```python
from build123d import *

# Parameters (mm, degrees)
SKETCH_R          = 1.6
PAD_DEPTH         = 6
SKETCH001_R       = 3
POCKET_DEPTH      = 40.001
POCKET_DEPTH_BACK = 40.001


with BuildPart() as toolbody:
    # Sketch → Pad (new body)
    with BuildSketch(Plane.XY):
        Polygon((46, -40), (0, -40), (0, -25), (17.5, -25), (0, -7.5), (0, 7.5), (0, 20), (10, 20), (10, 40), (46, 40), (56, 40), (56, -40), align=None)
        with Locations((53, 0)):
            Circle(SKETCH_R, mode=Mode.SUBTRACT)
        with Locations((53, 35)):
            Circle(SKETCH_R, mode=Mode.SUBTRACT)
        with Locations((53, -35)):
            Circle(SKETCH_R, mode=Mode.SUBTRACT)
        with Locations((39, 35)):
            Circle(SKETCH_R, mode=Mode.SUBTRACT)
        with Locations((39, 0)):
            Circle(SKETCH_R, mode=Mode.SUBTRACT)
        with Locations((39, -35)):
            Circle(SKETCH_R, mode=Mode.SUBTRACT)
        with Locations((15, 35)):
            Circle(SKETCH_R, mode=Mode.SUBTRACT)
        with Locations((15, -35)):
            Circle(SKETCH_R, mode=Mode.SUBTRACT)
        Polygon((15, 0), (28.75, 13.75), (28.75, -13.75), align=None, mode=Mode.SUBTRACT)
    extrude(amount=-PAD_DEPTH)

    # Sketch001 → Pocket (cut, two sides)
    with BuildSketch(Plane.XZ) as pocket_sk:
        with Locations((46, 0)):
            Circle(SKETCH001_R)
    extrude(amount=-POCKET_DEPTH, mode=Mode.SUBTRACT)
    extrude(pocket_sk.sketch, amount=POCKET_DEPTH_BACK, mode=Mode.SUBTRACT)


with BuildPart() as toolfusion:
    # Part__Mirroring: instance of ToolBody
    add(toolbody.part.mirror(Plane(origin=(0, 0, 0), x_dir=(0, -1, 0), z_dir=(1, 0, 0))))

    # Fusion: union ToolBody
    add(toolbody.part)


solid = toolfusion.part
```
Work out the finished part from the listing and answer in its coordinate system (mm). A direction names the side the tool comes from. Give positions to 0.01 mm unless a question says otherwise; leave off trailing zeros. Loops run counter-clockwise (first coordinate to the right, second up) from the corner with the lowest first, then second, coordinate; pieces in that order, holes last. Notation, with made-up numbers: M -33.5,56.5 L 13.5,56.5 A9 cw 13.5,68.5 Z; hole C 51,-5 d2. An arc over 180 degrees is marked long. One line per item, written item: value. Start each with the question number.
1. Find section B-B (x = -39). Give the vertices of the cut face in (y, z), and give its area (3 significant figures).
2. Which of the six approach directions +Z, -Z, +X, -X, +Y, -Y give full straight-line access (tool end or side, diameter ignored) to faces 3 (the face through (-22, -7, -3)), 4 (the face through (-46, 1, -3))?
3. Find section A-A (y = 8). Give the vertices of the cut face in (x, z).
4. Determine the mould class of faces 1 (the face through (37.82, 1.08, -2.96)), 2 (the face through (-51, 1, 0)) for opening direction X: released by +X, released by -X, zero draft, split by the parting line, or undercut.
5. Find section D-D (y = -5). Give the vertices of the cut face in (x, z), and give its area (3 significant figures).
6. Find the intervals of material crossed by probe 1 along Y at (x, z) = (-53, -2.85); probe 2 along Y at (x, z) = (25, -4.5); probe 3 along X at (y, z) = (12, -1.1), in increasing order.
7. Find section C-C (y = -31). Give the vertices of the cut face in (x, z).
8. Each of these flat-tipped pins is pushed along its axis until it touches: P1, Ø2.5, axis at x = -53, y = 0, coming from the -Z side; P2, Ø1.8, axis at x = -9, z = -3.5, coming from the +Y side. Where does it stop, or does it pass through?
Reported:
1. outline: M -40,-6 L -36.6,-6 L -36.6,0 L -40,0 Z; M -33.4,-6 L -1.6,-6 L -1.6,0 L -33.4,0 Z; M 1.6,-6 L 33.4,-6 L 33.4,0 L 1.6,0 Z; M 36.6,-6 L 40,-6 L 40,0 L 36.6,0 Z
1. area: 422 mm²
2. face 3: +Z, -Z
2. face 4: +Z, +Y, -Y
3. outline: M -56,-6 L -28.75,-6 L -28.75,0 L -43,0 A3 cw -49,0 L -56,0 Z; M -23,-6 L 23,-6 L 23,0 L -23,0 Z; M 28.75,-6 L 56,-6 L 56,0 L 49,0 A3 cw 43,0 L 28.75,0 Z
4. face 1: undercut
4. face 2: zero draft
5. outline: M -56,-6 L -28.75,-6 L -28.75,0 L -43,0 A3 cw -49,0 L -56,0 Z; M -20,-6 L 20,-6 L 20,0 L -20,0 Z; M 28.75,-6 L 56,-6 L 56,0 L 49,0 A3 cw 43,0 L 28.75,0 Z
5. area: 539 mm²
6. probe 1: y = -40 to -36.6, -33.4 to -1.6, 1.6 to 33.4, 36.6 to 40
6. probe 2: y = -40 to -10, 10 to 40
6. probe 3: x = -56 to -48.79, -43.21 to -28.75, -27 to 27, 28.75 to 43.21, 48.79 to 56
7. outline: M -56,-6 L 56,-6 L 56,0 L 49,0 A3 cw 43,0 L -43,0 A3 cw -49,0 L -56,0 Z
8. P1: passes through
8. P2: stops at y = 20
